from build123d import *

# Parameters (mm, degrees)
SKETCH2_W           = 50
SKETCH2_H           = 48
BOSS_EXTRUDE1_DEPTH = 1
CHAMFER1_SIZE       = 2
SKETCH3_R           = 1.6
SKETCH3_R_2         = 1.1
CUT_EXTRUDE1_DEPTH  = 35.713109915
SKETCH5_W           = 12
SKETCH5_H           = 12
BOSS_EXTRUDE2_DEPTH = 1.5
SKETCH6_W           = 6
SKETCH6_H           = 8
SKETCH6_H_2         = 10
BOSS_EXTRUDE3_DEPTH = 1.2


with BuildPart() as part:
    # Sketch2 → Boss-Extrude1 (new, symmetric)
    with BuildSketch(Plane(origin=(0, 0, 0), x_dir=(1, 0, 0), z_dir=(0, 1, 0))):
        Rectangle(SKETCH2_W, SKETCH2_H)
    extrude(amount=BOSS_EXTRUDE1_DEPTH, both=True)

    # Chamfer1
    chamfer1_edges = [part.edges().sort_by_distance(p)[0] for p in [
        (-25, 0, -24),
        (25, 0, -24),
        (25, 0, 24),
        (-25, 0, 24),
    ]]
    chamfer(chamfer1_edges, length=CHAMFER1_SIZE)

    # Sketch3 → Cut-Extrude1 (cut, through all)
    with BuildSketch(Plane(origin=(0, 1, 0), x_dir=(1, 0, 0), z_dir=(0, 1, 0))):
        with Locations(Location((-20, 21, 0), (0, 0, 270))):
            Circle(SKETCH3_R)
        with Locations(Location((20, 21, 0), (0, 0, 90))):
            Circle(SKETCH3_R)
        with Locations(Location((20, -21, 0), (0, 0, 270))):
            Circle(SKETCH3_R)
        with Locations(Location((-20, -21, 0), (0, 0, 90))):
            Circle(SKETCH3_R)
        with Locations(Location((0, 20, 0), (0, 0, 270))):
            Circle(SKETCH3_R_2)
        with Locations(Location((0, 2, 0), (0, 0, 270))):
            Circle(SKETCH3_R_2)
    extrude(amount=-CUT_EXTRUDE1_DEPTH, mode=Mode.SUBTRACT)

    # Sketch5 → Boss-Extrude2 (add)
    with BuildSketch(Plane(origin=(0, 1, 0), x_dir=(1, 0, 0), z_dir=(0, 1, 0))):
        with Locations((-14, -12)):
            Rectangle(SKETCH5_W, SKETCH5_H)
    extrude(amount=BOSS_EXTRUDE2_DEPTH)

    # Sketch6 → Boss-Extrude3 (add)
    with BuildSketch(Plane(origin=(0, 1, 0), x_dir=(1, 0, 0), z_dir=(0, 1, 0))):
        with Locations((-16, 12)):
            Rectangle(SKETCH6_W, SKETCH6_H)
        with Locations((12, -14)):
            Rectangle(SKETCH6_W, SKETCH6_H_2)
    extrude(amount=BOSS_EXTRUDE3_DEPTH)


solid = part.part
Verification items for the finished model (mm, model axes). A direction names the side the tool comes from. Coordinates: 2 decimals unless noted, no trailing zeros. Write each loop counter-clockwise with the first axis right and the second up, starting at its lowest first coordinate (ties: lowest second). Pieces come first, ordered by that corner, then holes. Notation, with made-up numbers: (-7.5, 64) - (25.5, 64) arc R29 cw to (25.5, 91) - close; hole circle Ø8 at (-39, 40). An arc over 180 degrees is marked (long way). Answer as a JSON object with one key per item and string values.
(1) Tool access check on faces 4 (the flat face through (12, 2, 9)), 5 (the flat face through (-20, 2, 12)), 6 (the flat face through (-16, 2.2, -12)). Record the directions out of +Z, -Z, +X, -X, +Y, -Y that give a thin tool (end or side, any length) a straight path to the whole face; none if there is none.
Report:
{"face 4": "-Z, +X, +Y", "face 5": "+Z, -Z, -X, +Y", "face 6": "-Z, +X, -X, +Y"}
(2) Cross-section at A-A on z = 21. Record the cut outline in (x, y).
Report:
{"outline": "(-25, -1) - (-21.6, -1) - (-21.6, 1) - (-25, 1) - close; (-18.4, -1) - (18.4, -1) - (18.4, 1) - (-18.4, 1) - close; (21.6, -1) - (25, -1) - (25, 1) - (21.6, 1) - close"}
(3) Cross-section at D-D on y = -0.45. Record the cut outline in (x, z).
Report:
{"outline": "(-25, -22) - (-23, -24) - (23, -24) - (25, -22) - (25, 22) - (23, 24) - (-23, 24) - (-25, 22) - close; hole circle Ø3.2 at (-20, -21); hole circle Ø3.2 at (-20, 21); hole circle Ø2.2 at (0, -20); hole circle Ø2.2 at (0, -2); hole circle Ø3.2 at (20, -21); hole circle Ø3.2 at (20, 21)"}
(4) Cross-section at B-B on x = 20. Record the cut outline in (y, z).
Report:
{"outline": "(-1, -24) - (1, -24) - (1, -22.6) - (-1, -22.6) - close; (-1, -19.4) - (1, -19.4) - (1, 19.4) - (-1, 19.4) - close; (-1, 22.6) - (1, 22.6) - (1, 24) - (-1, 24) - close"}
(5) Gauge pin test, flat ends, axial feed: pin 1 Ø1.8 at (x, z) = (11, 16) entering from +Y; pin 2 Ø14.5 at (x, z) = (5.5, 2) entering from +Y; pin 3 Ø0.6 at (x, y) = (10.5, 2) entering from +Z. Record the tip position at first contact, or that the pin passes through.
Report:
{"pin 1": "y = 2.2", "pin 2": "y = 1", "pin 3": "z = 19"}
(6) Mould release check, pull along X, two halves, no side actions. Record for faces 1 (the cylindrical face through (0, 0, -21.1)), 2 (the flat face through (-25, 0, 0)), 3 (the flat face through (-16, 2, -16)): pulls with the +X half, pulls with the -X half, needs draft (parallel to the pull), parting line crosses it, or undercut.
Report:
{"face 1": "undercut", "face 2": "pulls with the -X half", "face 3": "needs draft"}
(7) Cross-section at C-C on z = -2. Record the cut outline in (x, y).
Report:
{"outline": "(-25, -1) - (-1.1, -1) - (-1.1, 1) - (-25, 1) - close; (1.1, -1) - (25, -1) - (25, 1) - (1.1, 1) - close"}
(8) Thickness scan on line 1 along X through (y, z) = (-0.25, 21); line 2 along X through (y, z) = (0.2, -2); line 3 along X through (y, z) = (-0.45, -21). Record the ranges inside material, lowest first.
Report:
{"line 1": "-25 to -21.6, -18.4 to 18.4, 21.6 to 25", "line 2": "-25 to -1.1, 1.1 to 25", "line 3": "-25 to -21.6, -18.4 to -0.46, 0.46 to 18.4, 21.6 to 25"}
